Geometry check sheet. Reference: the model listing, model coordinates, mm. Round coordinates to 2 decimals unless told otherwise and drop trailing zeros. Loops run counter-clockwise (first coordinate to the right, second up) from the corner with the lowest first, then second, coordinate; pieces in that order, holes last.
```python
from build123d import *

# Parameters (mm, degrees)
SKETCH1_W           = 100
SKETCH1_H           = 140
SKETCH1_R           = 5.953762401
SKETCH1_R_2         = 2.054847291
SKETCH1_R_3         = 7.5
BOSS_EXTRUDE1_DEPTH = 6.35
FILLET1_R           = 2


with BuildPart() as part:
    # Sketch1 → Boss-Extrude1 (new body)
    with BuildSketch(Plane.XY):
        Rectangle(SKETCH1_W, SKETCH1_H)
        with Locations((-30.691299308, -50.95)):
            Circle(SKETCH1_R, mode=Mode.SUBTRACT)
        with Locations((30.040853965, -50.95)):
            Circle(SKETCH1_R, mode=Mode.SUBTRACT)
        with Locations((-41.650484861, 13.92267898)):
            Circle(SKETCH1_R_2, mode=Mode.SUBTRACT)
        with Locations((8.122482859, 61.869115774)):
            Circle(SKETCH1_R_2, mode=Mode.SUBTRACT)
        with Locations((35.06381401, 11.867831689)):
            Circle(SKETCH1_R_2, mode=Mode.SUBTRACT)
        with Locations((0, 30.582009883)):
            Circle(SKETCH1_R_3, mode=Mode.SUBTRACT)
    extrude(amount=BOSS_EXTRUDE1_DEPTH)

    # Fillet1
    fillet1_edges = [part.edges().sort_by_distance(p)[0] for p in [
        (50, -70, 3.175),
        (-50, -70, 3.175),
        (-50, 70, 3.175),
        (50, 70, 3.175),
    ]]
    fillet(fillet1_edges, radius=FILLET1_R)


solid = part.part
```
1) Sectioned sample at A-A, the plane y = -50.95. Record the cut outline in (x, z).
Report:
outline: (-50, 0) - (-36.65, 0) - (-36.65, 6.35) - (-50, 6.35) - close; (-24.74, 0) - (24.09, 0) - (24.09, 6.35) - (-24.74, 6.35) - close; (35.99, 0) - (50, 0) - (50, 6.35) - (35.99, 6.35) - close
2) Mould release check, pull along Y, two halves, no side actions. Record for faces 1 (the face through (-1, -70, 3)), 2 (the face through (7.855, 63.906, 3.131)), 3 (the face through (50, -1, 3)): +Y half, -Y half, draft (parallel to the pull), parting line (faces both ways), or undercut.
Report:
face 1: -Y half
face 2: undercut
face 3: draft
3) Sectioned sample at B-B, the plane x = 0. Record the cut outline in (y, z), then the cut area to 3 significant figures.
Report:
outline: (-70, 0) - (23.08, 0) - (23.08, 6.35) - (-70, 6.35) - close; (38.08, 0) - (70, 0) - (70, 6.35) - (38.08, 6.35) - close
area: 794 mm2
4) Scan lines: line 1 along Y through (x, z) = (0, 1.75); line 2 along X through (y, z) = (27, 1); line 3 along Y through (x, z) = (-40.5, 6). Record each from-to range of solid material in increasing order.
Report:
line 1: y = -70 to 23.08, 38.08 to 70
line 2: x = -50 to -6.59, 6.59 to 50
line 3: y = -70 to 12.22, 15.63 to 70
5) Sectioned sample at D-D, the plane x = 28.5. Record the cut outline in (y, z), then the cut area to 3 significant figures.
Report:
outline: (-70, 0) - (-56.7, 0) - (-56.7, 6.35) - (-70, 6.35) - close; (-45.2, 0) - (70, 0) - (70, 6.35) - (-45.2, 6.35) - close
area: 816 mm2
6) Sectioned sample at C-C, the plane z = 4. Record the cut outline in (x, y), then the cut area to 3 significant figures.
Report:
outline: (-50, -68) arc R2 ccw to (-48, -70) - (48, -70) arc R2 ccw to (50, -68) - (50, 68) arc R2 ccw to (48, 70) - (-48, 70) arc R2 ccw to (-50, 68) - close; hole circle Ø4.11 at (-41.65, 13.92); hole circle Ø11.91 at (-30.69, -50.95); hole circle Ø15 at (0, 30.58); hole circle Ø4.11 at (8.12, 61.87); hole circle Ø11.91 at (30.04, -50.95); hole circle Ø4.11 at (35.06, 11.87)
area: 13,600 mm2
